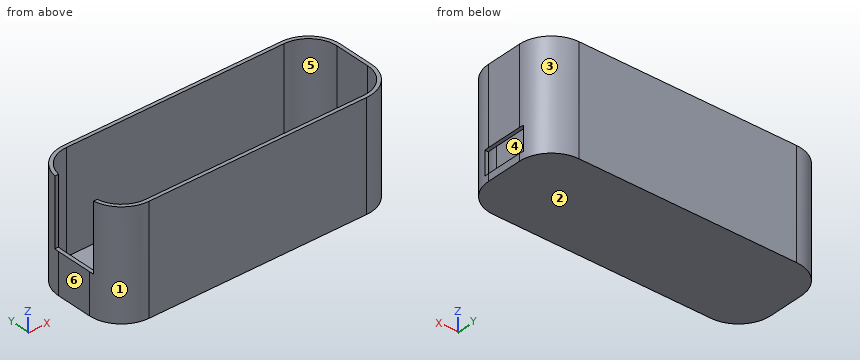
Autodesk Fusion 360 part; units mm, degrees
sketch "Sketch1" plane through (0, 0, 0) normal (0, 0, 1) x (1, 0, 0)
  line L0 (10, 0) -> (101.4, 0)
  line L1 (111.4, 10) -> (111.4, 25)
  line L2 (101.4, 35) -> (10, 35)
  line L3 (0, 25) -> (0, 10)
  arc A0 (10, 35) -> (0, 25) centre (10, 25) ccw
  arc A1 (0, 10) -> (10, 0) centre (10, 10) ccw
  arc A2 (101.4, 0) -> (111.4, 10) centre (101.4, 10) ccw
  arc A3 (111.4, 25) -> (101.4, 35) centre (101.4, 25) ccw
  line L4 (-2, 25) -> (-2, 10)
  arc A4 (-2, 10) -> (10, -2) centre (10, 10) ccw
  line L5 (10, -2) -> (101.4, -2)
  arc A5 (101.4, -2) -> (113.4, 10) centre (101.4, 10) ccw
  line L6 (113.4, 10) -> (113.4, 25)
  arc A6 (113.4, 25) -> (101.4, 37) centre (101.4, 25) ccw
  line L7 (101.4, 37) -> (10, 37)
  arc A7 (10, 37) -> (-2, 25) centre (10, 25) ccw
  line L8 (-3.5, 25) -> (-3.5, 10)
  arc A8 (-3.5, 10) -> (10, -3.5) centre (10, 10) ccw
  line L9 (10, -3.5) -> (101.4, -3.5)
  arc A9 (101.4, -3.5) -> (114.9, 10) centre (101.4, 10) ccw
  line L10 (114.9, 10) -> (114.9, 25)
  arc A10 (114.9, 25) -> (101.4, 38.5) centre (101.4, 25) ccw
  line L11 (101.4, 38.5) -> (10, 38.5)
  arc A11 (10, 38.5) -> (-3.5, 25) centre (10, 25) ccw
  point P0 (111.4, 0)
  point P1 (0, 35)
  dimension "d1" = 111.4
  dimension "d2" = 35
  dimension "d3" = 10
  dimension "d4" = 2
  dimension "d5" = 3.5
extrude "Extrude1" add sketch "Sketch1" along normal blind 3 contours L0 L1 L2 L3 A0 A1 A2 A3 | L4 A4 L5 A5 L6 A6 L7 A7 | L8 A8 L9 A9 L10 A10 L11 A11
extrude "Extrude2" add sketch "Sketch1" along normal blind 45 contours L8 A8 L9 A9 L10 A10 L11 A11
sketch "Sketch2" plane through (0, 0, 45) normal (0, 0, 1) x (-1, 0, 0)
  arc A0 (-10, -37) -> (2, -25) centre (-10, -25) ccw
  line L0 (-10, -37) -> (-101.4, -37)
  arc A1 (-113.4, -25) -> (-101.4, -37) centre (-101.4, -25) ccw
  line L1 (-113.4, -25) -> (-113.4, -10)
  arc A2 (-101.4, 2) -> (-113.4, -10) centre (-101.4, -10) ccw
  line L2 (-101.4, 2) -> (-10, 2)
  arc A3 (2, -10) -> (-10, 2) centre (-10, -10) ccw
  line L3 (2, -10) -> (2, -25)
  arc A4 (-10, -38.5) -> (3.5, -25) centre (-10, -25) ccw
  line L4 (3.5, -25) -> (3.5, -10)
  arc A5 (3.5, -10) -> (-10, 3.5) centre (-10, -10) ccw
  line L5 (-10, 3.5) -> (-101.4, 3.5)
  arc A6 (-101.4, 3.5) -> (-114.9, -10) centre (-101.4, -10) ccw
  line L6 (-114.9, -10) -> (-114.9, -25)
  arc A7 (-114.9, -25) -> (-101.4, -38.5) centre (-101.4, -25) ccw
  line L7 (-101.4, -38.5) -> (-10, -38.5)
  line L8 (2, -17.5) -> (2, -27) construction
  line L9 (2, -27) -> (1, -27) construction
  line L10 (1, -27) -> (11, -27)
  line L11 (11, -27) -> (11, -8)
  line L12 (11, -8) -> (1, -8)
  line L13 (1, -8) -> (1, -27)
  dimension "d12" = 9.5
  dimension "d13" = 1
  dimension "d14" = 19
extrude "Extrude5" cut sketch "Sketch2" against normal blind 28 contours A0 A3 L3 L10 L12 L13 | A0 A3 L3 A4 L4 A5 L10 L12 | A4 L4 A5 L10 L11 L12
sketch "Sketch3" plane through (114.9, 0, 0) normal (1, 0, 0) x (0, 1, 0)
  line L0 (10, 0) -> (25, 0)
  line L1 (25, 0) -> (25, 45)
  line L2 (25, 45) -> (10, 45)
  line L3 (10, 45) -> (10, 0)
  line L4 (17.5, 0) -> (17.5, 3) construction
  line L5 (17.5, 3) -> (27, 3) construction
  line L6 (27, 3) -> (8, 3)
  line L7 (8, 3) -> (8, 13)
  line L8 (8, 13) -> (27, 13)
  line L9 (27, 13) -> (27, 3)
  dimension "d19" = 3
  dimension "d20" = 9.5
  dimension "d21" = 19
  dimension "d22" = 10
extrude "Extrude6" cut sketch "Sketch3" against normal blind 10 contours L3 L6 L7 L8 | L1 L3 L6 L8 | L1 L6 L8 L9
Read the model definition and answer for the solid it produces. Units are mm, in the model's axes. Face numbers are marked on the shaded views. A direction names the side the tool comes from. Coordinates: 2 decimals unless noted, no trailing zeros. Loops run counter-clockwise (first coordinate to the right, second up) from the corner with the lowest first, then second, coordinate; pieces in that order, holes last. Notation, with made-up numbers: (72.5, 18.5) - (85.5, 18.5) arc R11 ccw to (85.5, 31.5) - close; hole circle Ø5 at (68, 42.25). An arc over 180 degrees is marked (long way). Answer in a Markdown table with one row per item.
1. Find section B-B, the plane z = 42. Write down the section's boundary in (x, y).
Conclusion:
| item | result |
|---|---|
| outline | (-3.35, 8) arc R13.5 ccw to (10, -3.5) - (101.4, -3.5) arc R13.5 ccw to (114.9, 10) - (114.9, 25) arc R13.5 ccw to (101.4, 38.5) - (10, 38.5) arc R13.5 ccw to (-3.35, 27) - (-1.83, 27) arc R12 cw to (10, 37) - (101.4, 37) arc R12 cw to (113.4, 25) - (113.4, 10) arc R12 cw to (101.4, -2) - (10, -2) arc R12 cw to (-1.83, 8) - close |
2. Straight lines are drawn through the part: line 1 (Y direction, x = 82, z = 7); line 2 (Z direction, x = 50.5, y = 15.5); line 3 (X direction, y = 15.5, z = 23.5). For each, find the intervals that lie inside material, in ascending order.
Conclusion:
| item | result |
|---|---|
| line 1 | y = -3.5 to -2, 37 to 38.5 |
| line 2 | z = 0 to 3 |
| line 3 | x = 113.4 to 114.9 |
3. Find section C-C, the plane x = 43.5. Write down the section's boundary in (y, z), then the cut area to 3 significant figures.
Conclusion:
| item | result |
|---|---|
| outline | (-3.5, 0) - (38.5, 0) - (38.5, 45) - (37, 45) - (37, 3) - (-2, 3) - (-2, 45) - (-3.5, 45) - close |
| area | 252 mm² |
4. Determine the mould class of the marked faces 1, 2, 3 and 4 for opening direction Y: +Y half, -Y half, draft (parallel to the pull), parting line (faces both ways), or undercut.
Conclusion:
| item | result |
|---|---|
| face 1 | -Y half |
| face 2 | draft |
| face 3 | +Y half |
| face 4 | undercut |
5. Which of the six approach directions +Z, -Z, +X, -X, +Y, -Y give full straight-line access (tool end or side, diameter ignored) to the marked faces 5 and 6?
Conclusion:
| item | result |
|---|---|
| face 5 | +Z |
| face 6 | +Z, -Z, -X, +Y, -Y |
6. Given pin 1 (3 mm diameter, centred on y = 28, z = 9, fed in from +X); pin 2 (0.5 mm diameter, centred on x = -2.5, z = 24, fed in from -Y); pin 3 (3 mm diameter, centred on x = 44, y = 22.5, fed in from +Z), each flat-ended and moving along its own axis, determine where each tip first touches the part or whether it passes through.
Conclusion:
| item | result |
|---|---|
| pin 1 | stops at x = 114.75 |
| pin 2 | stops at y = 4.33 |
| pin 3 | stops at z = 3 |
7. Find section A-A, the plane y = 18.5. Write down the section's boundary in (x, z), then the cut area to 3 significant figures.
Conclusion:
| item | result |
|---|---|
| outline | (-3.5, 0) - (114.9, 0) - (114.9, 3) - (-2, 3) - (-2, 17) - (-3.5, 17) - close; (113.4, 13) - (114.9, 13) - (114.9, 45) - (113.4, 45) - close |
| area | 424 mm² |
8. Find section D-D, the plane y = 35.5. Write down the section's boundary in (x, z).
Conclusion:
| item | result |
|---|---|
| outline | (1.51, 0) - (109.89, 0) - (109.89, 45) - (107.21, 45) - (107.21, 3) - (4.19, 3) - (4.19, 45) - (1.51, 45) - close |
